```python
from build123d import *

# Parameters (mm, degrees)
SKETCH1_R      = 15.98
EXTRUDE1_DEPTH = 15.2
SKETCH8_R      = 2
EXTRUDE3_DEPTH = 16.2
SKETCH9_R      = 2
EXTRUDE4_DEPTH = 16.2


with BuildPart() as part:
    # Sketch1 → Extrude1 (new body)
    with BuildSketch(Plane.XY):
        Circle(SKETCH1_R)
    extrude(amount=EXTRUDE1_DEPTH)

    # Sketch8 → Extrude3 (cut, through all)
    with BuildSketch(Plane.XY.offset(15.2)):
        Circle(SKETCH8_R)
    extrude(amount=-EXTRUDE3_DEPTH, mode=Mode.SUBTRACT)

    # Sketch9 → Extrude4 (cut, through all)
    with BuildSketch(Plane.XY.offset(15.2)):
        with Locations((0, 5)):
            Circle(SKETCH9_R)
    extrude(amount=-EXTRUDE4_DEPTH, mode=Mode.SUBTRACT)


solid = part.part
```
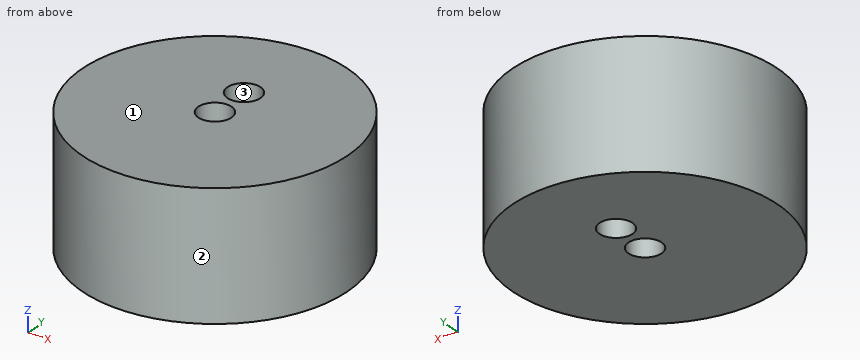
Could you check a few things on this model? Use its own coordinates, in mm. Face numbers are marked on the shaded views. Coordinates: 2 decimals unless noted, no trailing zeros. Loops run counter-clockwise (first coordinate to the right, second up) from the corner with the lowest first, then second, coordinate; pieces in that order, holes last.
1) Imagine slicing it at C-C (z = 13). List the corners of the cut face in (x, y) for me.
Reported:
outline: circle Ø31.96 at (0, 0); hole circle Ø4 at (0, 0); hole circle Ø4 at (0, 5)
2) Will these pins go through, and if not, where does the flat tip stop? pin 1 Ø3 at (y, z) = (-2, 12) entering from -X; pin 2 Ø3 at (x, z) = (4.5, 10.5) entering from -Y; pin 3 Ø8 at (y, z) = (-10.5, 1.5) entering from -X; pin 4 Ø2.5 at (x, y) = (0, 5) entering from +Z.
Reported:
pin 1: stops at x = -15.97
pin 2: stops at y = -15.7
pin 3: stops at x = -14.6
pin 4: passes through
3) Imagine slicing it at A-A (y = 0). List the corners of the cut face in (x, z) for me.
Reported:
outline: (-15.98, 0) - (-2, 0) - (-2, 15.2) - (-15.98, 15.2) - close; (2, 0) - (15.98, 0) - (15.98, 15.2) - (2, 15.2) - close
4) Imagine slicing it at D-D (y = 5). List the corners of the cut face in (x, z) for me.
Reported:
outline: (-15.18, 0) - (-2, 0) - (-2, 15.2) - (-15.18, 15.2) - close; (2, 0) - (15.18, 0) - (15.18, 15.2) - (2, 15.2) - close
5) Please list where these lines run through material, in increasing order: line 1 along Y through (x, z) = (0, 7.5); line 2 along X through (y, z) = (-1, 2.5); line 3 along X through (y, z) = (-4.5, 10.5).
Reported:
line 1: y = -15.98 to -2, 2 to 3, 7 to 15.98
line 2: x = -15.95 to -1.73, 1.73 to 15.95
line 3: x = -15.33 to 15.33
6) Thinking about a two-plate mould opening in Y: for the marked faces 1, 2 and 3, which applies, released by +Y, released by -Y, zero draft, split by the parting line, or undercut?
Reported:
face 1: zero draft
face 2: split by the parting line
face 3: undercut
7) Imagine slicing it at B-B (x = 0). List the corners of the cut face in (y, z) for me, and give its area (3 significant figures).
Reported:
outline: (-15.98, 0) - (-2, 0) - (-2, 15.2) - (-15.98, 15.2) - close; (2, 0) - (3, 0) - (3, 15.2) - (2, 15.2) - close; (7, 0) - (15.98, 0) - (15.98, 15.2) - (7, 15.2) - close
area: 364 mm2
